Work out the finished part from the listing and answer in its coordinate system (mm). A direction names the side the tool comes from. Give positions to 0.01 mm unless a question says otherwise; leave off trailing zeros. Loops run counter-clockwise (first coordinate to the right, second up) from the corner with the lowest first, then second, coordinate; pieces in that order, holes last. Notation, with made-up numbers: (-14, 81) - (3, 81) arc R33 cw to (3, 118) - close; hole circle Ø3 at (22.5, -28). An arc over 180 degrees is marked (long way). One line per question, with ' | ' between items. Start each with the question number.
1. For a pull along X with two mould halves and no side action, classify faces 1 (the face through (-6, 1, 2)), 2 (the face through (-2.3, 1.8, 2)), 3 (the face through (-0.777, 1.76, 1.972)), 4 (the face through (0, 1, 2)) as released by +X, released by -X, zero draft, split by the parting line, or undercut.
2. Section D-D (y = 0.6) is taken. Determine the outline of the cut face in (x, z).
3. Section B-B (y = 2) is taken. Determine the outline of the cut face in (x, z), plus the area to 3 significant figures.
4. Which of the six approach directions +Z, -Z, +X, -X, +Y, -Y give full straight-line access (tool end or side, diameter ignored) to faces 5 (the face through (-6.244, 0.715, 0.301)), 6 (the face through (2, 2.5, 2)), 7 (the face through (2.723, 1.76, 1.972))?
5. This flat-tipped pin is pushed along its axis until it touches: pin 1 (0.7 mm diameter, centred on x = 7.5, z = 2, fed in from +Y). Where does it stop, or does it pass through?
6. Find the intervals of material crossed by line 1 (X direction, y = 1.9, z = 3.2); line 2 (X direction, y = 2.35, z = 0.2); line 3 (Z direction, x = -9, y = 0.1) (3 decimals), in increasing order.
7. Section C-C (x = 6.75) is taken. Determine the outline of the cut face in (y, z), plus the area to 3 significant figures.
8. Section A-A (z = 1.65) is taken. Determine the outline of the cut face in (x, y).
from build123d import *

# Parameters (mm, degrees)
BOSS_EXTRUDE1_DEPTH = 4
FILLET1_R           = 1


with BuildPart() as part:
    # Sketch1 → Boss-Extrude1 (new body)
    with BuildSketch(Plane.XY):
        Polygon((6.5, 1), (7.908089297, 1), (8.454044649, 2.5), (9.454044649, 2.5), (10, 1), (10, -1), (-10, -1), (-10, 1), (-2.591910703, 1), (-2.045955351, 2.5), (-1.045955351, 2.5), (-0.5, 1), (0.908089297, 1), (1.454044649, 2.5), (2.454044649, 2.5), (3, 1), (4.408089297, 1), (4.954044649, 2.5), (5.954044649, 2.5), align=None)
    extrude(amount=BOSS_EXTRUDE1_DEPTH)

    # Fillet1
    fillet1_edges = [part.edges().sort_by_distance(p)[0] for p in [
        (0, -1, 4),
        (0, -1, 0),
        (-6.295955351, 1, 0),
        (-6.295955351, 1, 4),
    ]]
    fillet(fillet1_edges, radius=FILLET1_R - 0.0001)  # a hair under: the kernel refuses the full size


solid = part.part
Conclusion:
1) face 1: zero draft | face 2: released by -X | face 3: undercut | face 4: undercut
2) outline: (-10, 0.2) - (-2.74, 0.2) - (-2.74, 0) - (10, 0) - (10, 4) - (-2.74, 4) - (-2.74, 3.8) - (-10, 3.8) - close
3) outline: (-2.23, 0) - (-0.86, 0) - (-0.86, 4) - (-2.23, 4) - close; (1.27, 0) - (2.64, 0) - (2.64, 4) - (1.27, 4) - close; (4.77, 0) - (6.14, 0) - (6.14, 4) - (4.77, 4) - close; (8.27, 0) - (9.64, 0) - (9.64, 4) - (8.27, 4) - close | area: 21.8 mm²
4) face 5: -Z, -X, +Y | face 6: +Z, -Z, +X, -X, +Y | face 7: +Z, -Z, +Y
5) pin 1: y = 1
6) line 1: -2.26 to -0.83, 1.24 to 2.67, 4.74 to 6.17, 8.24 to 9.67 | line 2: -2.1 to -0.99, 1.4 to 2.51, 4.9 to 6.01, 8.4 to 9.51 | line 3: 0.005 to 3.995
7) outline: (-1, 1) arc R1 ccw to (0, 0) - (1, 0) - (1, 4) - (0, 4) arc R1 ccw to (-1, 3) - close | area: 7.57 mm²
8) outline: (-10, -1) - (10, -1) - (10, 1) - (9.45, 2.5) - (8.45, 2.5) - (7.91, 1) - (6.5, 1) - (5.95, 2.5) - (4.95, 2.5) - (4.41, 1) - (3, 1) - (2.45, 2.5) - (1.45, 2.5) - (0.91, 1) - (-0.5, 1) - (-1.05, 2.5) - (-2.05, 2.5) - (-2.59, 1) - (-10, 1) - close
